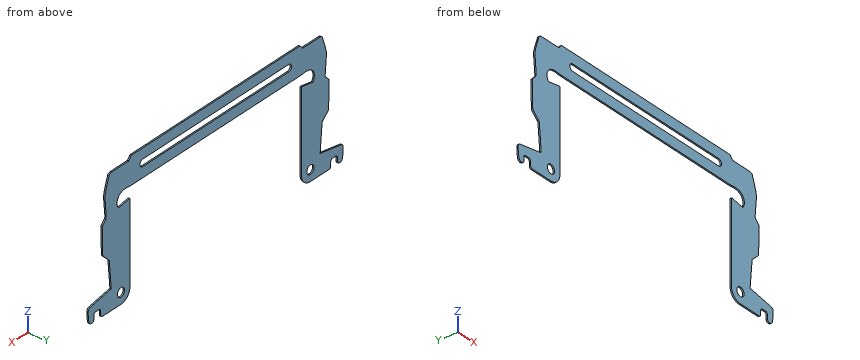
Autodesk Inventor part; units mm, degrees
ref_plane "YZ Plane" through (0, 0, 0) normal (1, 0, 0) x (0, 1, 0)
ref_plane "XZ Plane" through (0, 0, 0) normal (0, 1, 0) x (-1, 0, 0)
ref_plane "XY Plane" through (0, 0, 0) normal (0, 0, 1) x (1, 0, 0)
sketch "Эскиз1" plane through (0, 0, 0) normal (0, 1, 0) x (-1, 0, 0)
  circle A0 centre (-4.631, -43.5563) radius 1.6
  arc A1 (5, -3.75) -> (5, -6.25) centre (5, -5) ccw
  line L0 (5, -3.75) -> (70, -3.75)
  arc A2 (70, -6.25) -> (70, -3.75) centre (70, -5) ccw
  line L1 (70, -6.25) -> (5, -6.25)
  arc A3 (77.3239, -9.8413) -> (76.131, -9.9442) centre (79.631, -43.5563) ccw
  arc A4 (79.4677, -10.1658) -> (77.3239, -9.8413) centre (77.6653, -14.8296) ccw
  arc A5 (80.6854, -14.8912) -> (79.4677, -10.1658) centre (78.3862, -12.9641) ccw
  line L2 (80.6854, -14.8912) -> (75.8657, -14.0414)
  arc A6 (75.8657, -14.0414) -> (75.631, -14.2384) centre (75.831, -14.2384) ccw
  line L3 (75.631, -14.2384) -> (75.631, -43.5563)
  arc A7 (75.631, -43.5563) -> (79.631, -47.5563) centre (79.631, -43.5563) ccw
  line L4 (79.631, -47.5563) -> (87.8552, -47.5563)
  arc A8 (87.8552, -47.5563) -> (88.6552, -46.7563) centre (87.8552, -46.7563) ccw
  line L5 (88.6552, -46.7563) -> (88.6552, -45.3563)
  arc A9 (89.4552, -44.5563) -> (88.6552, -45.3563) centre (89.4552, -45.3563) ccw
  line L6 (89.4552, -44.5563) -> (90.8552, -44.5563)
  arc A10 (91.6552, -45.3563) -> (90.8552, -44.5563) centre (90.8552, -45.3563) ccw
  line L7 (91.6552, -45.3563) -> (91.6552, -46.7563)
  arc A11 (91.6552, -46.7563) -> (92.4552, -47.5563) centre (92.4552, -46.7563) ccw
  line L8 (92.4552, -47.5563) -> (92.8552, -47.5563)
  arc A12 (92.8552, -47.5563) -> (93.8304, -46.7775) centre (92.8552, -46.5563) ccw
  arc A13 (93.8304, -46.7775) -> (94.174, -42.8497) centre (79.631, -43.5563) ccw
  arc A14 (94.174, -42.8497) -> (93.3489, -41.9134) centre (93.1752, -42.8982) ccw
  line L9 (93.3489, -41.9134) -> (83.9409, -40.2546)
  line L10 (83.9409, -40.2546) -> (84.7989, -30.6198)
  arc A15 (85.1049, -29.9847) -> (84.7989, -30.6198) centre (85.795, -30.7085) ccw
  line L11 (85.1049, -29.9847) -> (87.4169, -27.7806)
  arc A16 (87.4169, -27.7806) -> (87.7266, -27.0807) centre (86.7269, -27.0568) ccw
  line L12 (87.7266, -27.0807) -> (87.9456, -17.9117)
  arc A17 (87.9456, -17.9117) -> (87.6697, -17.1978) centre (86.9459, -17.8878) ccw
  line L13 (87.6697, -17.1978) -> (86.4498, -15.9183)
  arc A18 (86.1776, -15.1396) -> (86.4498, -15.9183) centre (87.1736, -15.2283) ccw
  line L14 (86.1776, -15.1396) -> (86.7309, -8.9267)
  arc A19 (86.7309, -8.9267) -> (86.6462, -7.4668) centre (81.7506, -8.4832) ccw
  arc A20 (86.6462, -7.4668) -> (86.0376, -5.2239) centre (67.7491, -11.39) ccw
  line L15 (86.0376, -5.2239) -> (84.9746, -2.0709)
  arc A21 (84.9746, -2.0709) -> (84.1332, -1.396) centre (84.027, -2.3904) ccw
  arc A22 (84.1332, -1.396) -> (83.7286, -1.3548) centre (79.631, -43.5563) ccw
  arc A23 (83.7286, -1.3548) -> (83.5353, -1.3454) centre (83.5353, -3.3454) ccw
  line L16 (83.5353, -1.3454) -> (76.131, -1.3454)
  line L17 (76.131, -1.3454) -> (75, 0)
  line L18 (0, 0) -> (75, 0)
  line L19 (-1.131, -1.3454) -> (0, 0)
  line L20 (-8.5353, -1.3454) -> (-1.131, -1.3454)
  arc A24 (-8.5353, -1.3454) -> (-8.7286, -1.3548) centre (-8.5353, -3.3454) ccw
  arc A25 (-8.7286, -1.3548) -> (-9.1332, -1.396) centre (-4.631, -43.5563) ccw
  arc A26 (-9.1332, -1.396) -> (-9.9746, -2.0709) centre (-9.027, -2.3904) ccw
  line L21 (-11.0376, -5.2239) -> (-9.9746, -2.0709)
  arc A27 (-11.0376, -5.2239) -> (-11.6462, -7.4668) centre (7.2509, -11.39) ccw
  arc A28 (-11.6462, -7.4668) -> (-11.7309, -8.9267) centre (-6.7506, -8.4832) ccw
  line L22 (-11.1776, -15.1396) -> (-11.7309, -8.9267)
  arc A29 (-11.4498, -15.9183) -> (-11.1776, -15.1396) centre (-12.1736, -15.2283) ccw
  line L23 (-12.6697, -17.1978) -> (-11.4498, -15.9183)
  arc A30 (-12.6697, -17.1978) -> (-12.9456, -17.9117) centre (-11.9459, -17.8878) ccw
  line L24 (-12.7266, -27.0807) -> (-12.9456, -17.9117)
  arc A31 (-12.7266, -27.0807) -> (-12.4169, -27.7806) centre (-11.7269, -27.0568) ccw
  line L25 (-10.1049, -29.9847) -> (-12.4169, -27.7806)
  arc A32 (-9.7989, -30.6198) -> (-10.1049, -29.9847) centre (-10.795, -30.7085) ccw
  line L26 (-8.9409, -40.2546) -> (-9.7989, -30.6198)
  line L27 (-18.3489, -41.9134) -> (-8.9409, -40.2546)
  arc A33 (-18.3489, -41.9134) -> (-19.174, -42.8497) centre (-18.1752, -42.8982) ccw
  arc A34 (-19.174, -42.8497) -> (-18.8304, -46.7775) centre (-4.631, -43.5563) ccw
  arc A35 (-18.8304, -46.7775) -> (-17.8552, -47.5563) centre (-17.8552, -46.5563) ccw
  line L28 (-17.4552, -47.5563) -> (-17.8552, -47.5563)
  arc A36 (-17.4552, -47.5563) -> (-16.6552, -46.7563) centre (-17.4552, -46.7563) ccw
  line L29 (-16.6552, -45.3563) -> (-16.6552, -46.7563)
  arc A37 (-15.8552, -44.5563) -> (-16.6552, -45.3563) centre (-15.8552, -45.3563) ccw
  line L30 (-14.4552, -44.5563) -> (-15.8552, -44.5563)
  arc A38 (-13.6552, -45.3563) -> (-14.4552, -44.5563) centre (-14.4552, -45.3563) ccw
  line L31 (-13.6552, -46.7563) -> (-13.6552, -45.3563)
  arc A39 (-13.6552, -46.7563) -> (-12.8552, -47.5563) centre (-12.8552, -46.7563) ccw
  line L32 (-4.631, -47.5563) -> (-12.8552, -47.5563)
  arc A40 (-4.631, -47.5563) -> (-0.631, -43.5563) centre (-4.631, -43.5563) ccw
  line L33 (-0.631, -14.2384) -> (-0.631, -43.5563)
  arc A41 (-0.631, -14.2384) -> (-0.8657, -14.0414) centre (-0.831, -14.2384) ccw
  line L34 (-5.6854, -14.8912) -> (-0.8657, -14.0414)
  arc A42 (-4.4677, -10.1658) -> (-5.6854, -14.8912) centre (-3.3862, -12.9641) ccw
  arc A43 (-2.3239, -9.8413) -> (-4.4677, -10.1658) centre (-2.6653, -14.8296) ccw
  arc A44 (-1.131, -9.9442) -> (-2.3239, -9.8413) centre (-4.631, -43.5563) ccw
  line L35 (0, -10) -> (-1.131, -9.9442)
  line L36 (75, -10) -> (0, -10)
  line L37 (75, -10) -> (76.131, -9.9442)
  circle A45 centre (79.631, -43.5563) radius 1.6
extrude "Выдавливание1" add sketch "Эскиз1" along normal blind 0.5
properties part number "petal_forPrint"
Can you work these out from the model? Positions are in its coordinate system, mm. Give positions to 0.01 mm unless a question says otherwise; leave off trailing zeros. Loops run counter-clockwise (first coordinate to the right, second up) from the corner with the lowest first, then second, coordinate; pieces in that order, holes last. Notation, with made-up numbers: (0.5, -7.75) -> (22.5, -7.75) arc R10 cw to (22.5, -3.75) -> close; hole circle Ø11 at (16.5, 88). An arc over 180 degrees is marked (long way). Return JSON: item names as keys, results as strings.
Q1. I need wall thicknesses on probe 1 along X at (y, z) = (0.15, -21.5); probe 2 along Z at (x, y) = (-63.5, 0.25); probe 3 along Z at (x, y) = (-81, 0.45). Which ranges of each line are inside material? Lowest first, please.
Checks:
{"probe 1": "x = -87.86 to -75.63, 0.63 to 12.86", "probe 2": "z = -10 to -6.25, -3.75 to 0", "probe 3": "z = -47.56 to -44.38, -42.73 to -14.44, -11.49 to -1.35"}
Q2. I want a section at C-C, the plane y = 0.1. Count the separate pieces of the cut face and the enclosed holes in it, then the cut area to 3 significant figures.
Checks:
{"separate pieces": "1", "enclosed holes": "3", "area": "1,580 mm2"}
Q3. I want a section at B-B, the plane z = -22.5. List the corners of the cut face in (x, y) for me.
Checks:
{"outline": "(-87.84, 0) -> (-75.63, 0) -> (-75.63, 0.5) -> (-87.84, 0.5) -> close; (0.63, 0) -> (12.84, 0) -> (12.84, 0.5) -> (0.63, 0.5) -> close"}
Q4. I want a section at A-A, the plane x = -61.5. List the corners of the cut face in (y, z) for me, then the cut area to 3 significant figures.
Checks:
{"outline": "(0, -10) -> (0.5, -10) -> (0.5, -6.25) -> (0, -6.25) -> close; (0, -3.75) -> (0.5, -3.75) -> (0.5, 0) -> (0, 0) -> close", "area": "3.75 mm2"}
